Verification items for the finished model (mm, model axes). A direction names the side the tool comes from. Round coordinates to 2 decimals unless told otherwise and drop trailing zeros. Order: outer loops, then holes, each group sorted by start corner. A loop starts at its lowest first (then second) coordinate and runs counter-clockwise, first axis right, second up.
Autodesk Inventor part; units mm, degrees
ref_plane "YZ Plane" through (0, 0, 0) normal (1, 0, 0) x (0, 1, 0)
ref_plane "XZ Plane" through (0, 0, 0) normal (0, 1, 0) x (-1, 0, 0)
ref_plane "XY Plane" through (0, 0, 0) normal (0, 0, 1) x (1, 0, 0)
sketch "Esquisse1" plane through (0, 0, 0) normal (0, 0, 1) x (1, 0, 0)
  line L0 (0, 25) -> (65, 25)
  line L1 (65, 25) -> (65, 0)
  line L2 (65, 0) -> (0, 0)
  line L3 (0, 0) -> (0, 25)
  line L4 (-13, 0) -> (78, 0)
  line L5 (0, -5) -> (0, 30)
  point P0 (0, 0)
  dimension "d0" = 25
  dimension "d1" = 65
extrude "Extrusion1" add sketch "Esquisse1" along normal blind 2
sketch "Esquisse2" plane through (0, 0, 2) normal (0, 0, 1) x (1, 0, 0)
  line L0 (19, 24) -> (46, 24)
  line L1 (46, 24) -> (46, 10)
  line L2 (46, 10) -> (19, 10)
  line L3 (19, 10) -> (19, 24)
  line L4 (65, 0) -> (65, 25)
  line L5 (65, 25) -> (0, 25)
  line L6 (0, 0) -> (65, 0)
  dimension "d4" = 27
  dimension "d6" = 19
  dimension "d11" = 10
  dimension "d12" = 1
extrude "Extrusion2" add sketch "Esquisse2" along normal blind 6
sketch "Esquisse3" plane through (0, 0, 2) normal (0, 0, 1) x (1, 0, 0)
  line L0 (6, 9) -> (19, 9)
  line L1 (19, 9) -> (19, -1)
  line L2 (19, -1) -> (6, -1)
  line L3 (6, -1) -> (6, 9)
  line L4 (0, 25) -> (0, 0)
  line L5 (0, 0) -> (65, 0)
  line L6 (22, 9) -> (35, 9)
  line L7 (35, 9) -> (35, -1)
  line L8 (35, -1) -> (22, -1)
  line L9 (22, -1) -> (22, 9)
  dimension "d10" = 10
  dimension "d13" = 13
  dimension "d14" = 6
  dimension "d15" = 1
  dimension "d16" = 10
  dimension "d17" = 13
  dimension "d18" = 3
  dimension "d19" = 1
extrude "Extrusion3" add sketch "Esquisse3" along normal blind 7
equation "\"d16\" = d10"
equation "\"d17\" = d13"
equation "\"d19\" = d15"
properties part number "Power"
1) Sectioned sample at D-D on y = 14.5. Record the cut outline in (x, z), then the cut area to 3 significant figures.
2) Draft check along X on faces 1 (the flat face through (12, 4, 9)), 2 (the flat face through (35, 4, 5)), 3 (the flat face through (22, 4, 5)). Enter one of: released by +X, released by -X, zero draft, split by the parting line, or undercut.
3) Scan lines: probe 1 along Y at (x, z) = (25, 2.25); probe 2 along X at (y, z) = (0.5, 8.75); probe 3 along Z at (x, y) = (44, 21). Record each from-to range of solid material in increasing order.
4) Sectioned sample at A-A on z = 6.25. Record the cut outline in (x, y).
5) Tool access check on faces 4 (the flat face through (12, 9, 5)), 5 (the flat face through (33, 0, 1)), 6 (the flat face through (28, 9, 5)), 7 (the flat face through (19, 4, 5)). Record the directions out of +Z, -Z, +X, -X, +Y, -Y that give a thin tool (end or side, any length) a straight path to the whole face; none if there is none.
6) Sectioned sample at C-C on x = 40.5. Record the cut outline in (y, z), then the cut area to 3 significant figures.
7) Go/stop test with flat-tipped pins: pin 1 Ø8 at (x, y) = (51.5, 21) entering from +Z; pin 2 Ø1.8 at (y, z) = (14, 5) entering from -X; pin 3 Ø1.8 at (x, z) = (35.5, 6) entering from +Y. Record where each tip stops, or that it passes through.
8) Sectioned sample at B-B on y = 3. Record the cut outline in (x, z), then the cut area to 3 significant figures.
Returned:
1. outline: (0, 0) - (65, 0) - (65, 2) - (46, 2) - (46, 8) - (19, 8) - (19, 2) - (0, 2) - close
1. area: 292 mm2
2. face 1: zero draft
2. face 2: released by +X
2. face 3: undercut
3. probe 1: y = -1 to 9, 10 to 24
3. probe 2: x = 6 to 19, 22 to 35
3. probe 3: z = 0 to 8
4. outline: (6, -1) - (19, -1) - (19, 9) - (6, 9) - close; (19, 10) - (46, 10) - (46, 24) - (19, 24) - close; (22, -1) - (35, -1) - (35, 9) - (22, 9) - close
5. face 4: +Z, +X, -X, +Y
5. face 5: -Z, +X, -X, -Y
5. face 6: +Z, +X, -X
5. face 7: +Z, -Y
6. outline: (0, 0) - (25, 0) - (25, 2) - (24, 2) - (24, 8) - (10, 8) - (10, 2) - (0, 2) - close
6. area: 134 mm2
7. pin 1: stops at z = 2
7. pin 2: stops at x = 19
7. pin 3: stops at y = 24
8. outline: (0, 0) - (65, 0) - (65, 2) - (35, 2) - (35, 9) - (22, 9) - (22, 2) - (19, 2) - (19, 9) - (6, 9) - (6, 2) - (0, 2) - close
8. area: 312 mm2
